Could you check a few things on this model? Use its own coordinates, in mm. Face numbers are marked on the shaded views. A direction names the side the tool comes from. Give positions to 0.01 mm unless a question says otherwise; leave off trailing zeros. Order: outer loops, then holes, each group sorted by start corner. A loop starts at its lowest first (then second) coordinate and runs counter-clockwise, first axis right, second up. Notation, with made-up numbers: (62.5, -14) - (109.5, -14) arc R7 cw to (109.5, -10) - close; hole circle Ø5 at (41, -4). An arc over 180 degrees is marked (long way). Put each result on its own line as item: value.
from build123d import *

# Parameters (mm, degrees)
CROQUIS1_R              = 4
SALIENTE_EXTRUIR1_DEPTH = 52
CROQUIS2_R              = 5
SALIENTE_EXTRUIR2_DEPTH = 5
CROQUIS3_R              = 4
CROQUIS3_R_2            = 3
CORTAR_EXTRUIR1_DEPTH   = 22
CROQUIS5_R              = 1.25
CORTAR_EXTRUIR2_DEPTH   = 54.009433123
CHAFL_N1_SIZE           = 0.5
CROQUIS6_W              = 6
CROQUIS6_H              = 6
CORTAR_EXTRUIR3_DEPTH   = 53.775467786
CROQUIS7_R              = 4
CROQUIS7_R_2            = 3.25
CORTAR_EXTRUIR4_DEPTH   = 8
REDONDEO2_R             = 0.15
REDONDEO3_R             = 0.2
REDONDEO1_R             = 0.3
REDONDEO4_R             = 0.3
REDONDEO5_R             = 0.3


with BuildPart() as part:
    # Croquis1 → Saliente-Extruir1 (new, symmetric)
    with BuildSketch(Plane.XY):
        with Locations(Location((0, 0, 0), (0, 0, 180))):
            Circle(CROQUIS1_R)
    extrude(amount=SALIENTE_EXTRUIR1_DEPTH, both=True)

    # Croquis2 → Saliente-Extruir2 (add)
    with BuildSketch(Plane.XY.offset(-28.5)):
        Circle(CROQUIS2_R)
    extrude(amount=SALIENTE_EXTRUIR2_DEPTH)

    # Croquis3 → Cortar-Extruir1 (cut)
    with BuildSketch(Plane.XY.offset(52)):
        with Locations(Location((0, 0, 0), (0, 0, 180))):
            Circle(CROQUIS3_R)
        Circle(CROQUIS3_R_2, mode=Mode.SUBTRACT)
    extrude(amount=-CORTAR_EXTRUIR1_DEPTH, mode=Mode.SUBTRACT)

    # Croquis5 → Cortar-Extruir2 (cut, through all)
    with BuildSketch(Plane(origin=(0, 4, 0), x_dir=(1, 0, 0), z_dir=(0, 1, 0))):
        with Locations(Location((0, 41.5, 0), (0, 0, 270))):
            Circle(CROQUIS5_R)
    extrude(amount=-CORTAR_EXTRUIR2_DEPTH, mode=Mode.SUBTRACT)

    # Chaflán1
    chafl_n1_edges = [part.edges().sort_by_distance(p)[0] for p in [
        (-3, 0, 52),
        (4, 0, -52),
    ]]
    chamfer(chafl_n1_edges, length=CHAFL_N1_SIZE)

    # Croquis6 → Cortar-Extruir3 (cut, through all)
    with BuildSketch(Plane(origin=(0, 2.5, 0), x_dir=(1, 0, 0), z_dir=(0, 1, 0))):
        with Locations((0, -49)):
            Rectangle(CROQUIS6_W, CROQUIS6_H)
    extrude(amount=CORTAR_EXTRUIR3_DEPTH, mode=Mode.SUBTRACT)

    # Croquis7 → Cortar-Extruir4 (cut)
    with BuildSketch(Plane.XY.offset(30)):
        with Locations(Location((0, 0, 0), (0, 0, 180))):
            Circle(CROQUIS7_R)
        Circle(CROQUIS7_R_2, mode=Mode.SUBTRACT)
    extrude(amount=-CORTAR_EXTRUIR4_DEPTH, mode=Mode.SUBTRACT)

    # Redondeo2
    redondeo2_edges = [part.edges().sort_by_distance(p)[0] for p in [
        (-3, 0, 30),
    ]]
    fillet(redondeo2_edges, radius=REDONDEO2_R)

    # Redondeo3
    redondeo3_edges = [part.edges().sort_by_distance(p)[0] for p in [
        (-3.25, 0, 22),
    ]]
    fillet(redondeo3_edges, radius=REDONDEO3_R)

    # Redondeo1
    redondeo1_edges = [part.edges().sort_by_distance(p)[0] for p in [
        (4, 0, -23.5),
    ]]
    fillet(redondeo1_edges, radius=REDONDEO1_R)

    # Redondeo4
    redondeo4_edges = [part.edges().sort_by_distance(p)[0] for p in [
        (4, 0, -28.5),
    ]]
    fillet(redondeo4_edges, radius=REDONDEO4_R)

    # Redondeo5
    redondeo5_edges = [part.edges().sort_by_distance(p)[0] for p in [
        (0, 2.5, 46),
    ]]
    fillet(redondeo5_edges, radius=REDONDEO5_R)


solid = part.part
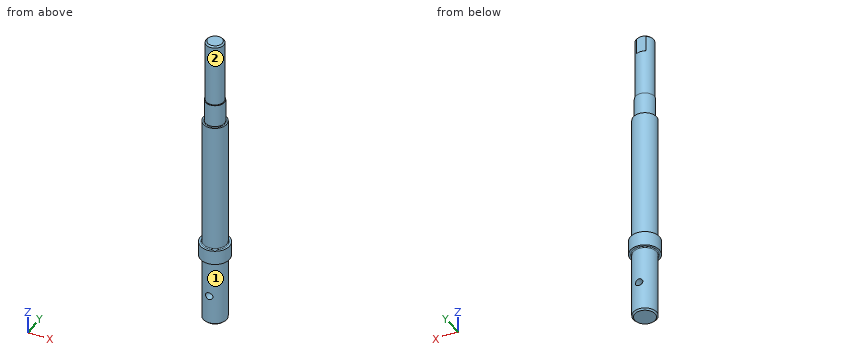
1) I'm going to push flat-ended pins straight in: pin 1 (3 mm diameter, centred on x = -0.5, z = -32.5, fed in from +Y); pin 2 (2 mm diameter, centred on x = -1.5, z = -24, fed in from -Y); pin 3 (1 mm diameter, centred on x = 0.5, z = 50.5, fed in from +Y). Where does each tip first touch, or does it pass through?
Filled in:
pin 1: stops at y = 4
pin 2: stops at y = -4.97
pin 3: stops at y = 2.5
2) Suppose I cut it at D-D, the plane z = 27.5. List the corners of the cut face in (x, y) for me.
Filled in:
outline: circle Ø6.5 at (0, 0)
3) Which directions (+Z, -Z, +X, -X, +Y, -Y) give clear straight access to the entire face, cutting with the end or side of a thin tool? Please do the marked faces 1 and 2.
Filled in:
face 1: -Z
face 2: +Z
4) Suppose I cut it at B-B, the plane z = 7. List the corners of the cut face in (x, y) for me, and give its area (3 significant figures).
Filled in:
outline: circle Ø8 at (0, 0)
area: 50.3 mm^2
5) Suppose I cut it at C-C, the plane z = -41.5. List the corners of the cut face in (x, y) for me.
Filled in:
outline: (-1.25, -3.8) - (-1.25, 3.8) arc R4 ccw to start; (1.25, -3.8) arc R4 ccw to (1.25, 3.8) - close
6) If I drill on line 1 (X direction, y = 0.25, z = -41.5); line 2 (Z direction, x = 0, y = -2); line 3 (Y direction, x = 0, z = -10.5), over which ranges is the centre line in solid material (lowest first)? Write a range as [from, to].
Filled in:
line 1: x = [-3.99, -1.25], [1.25, 3.99]
line 2: z = [-52, -42.75], [-40.25, 52]
line 3: y = [-4, 4]
